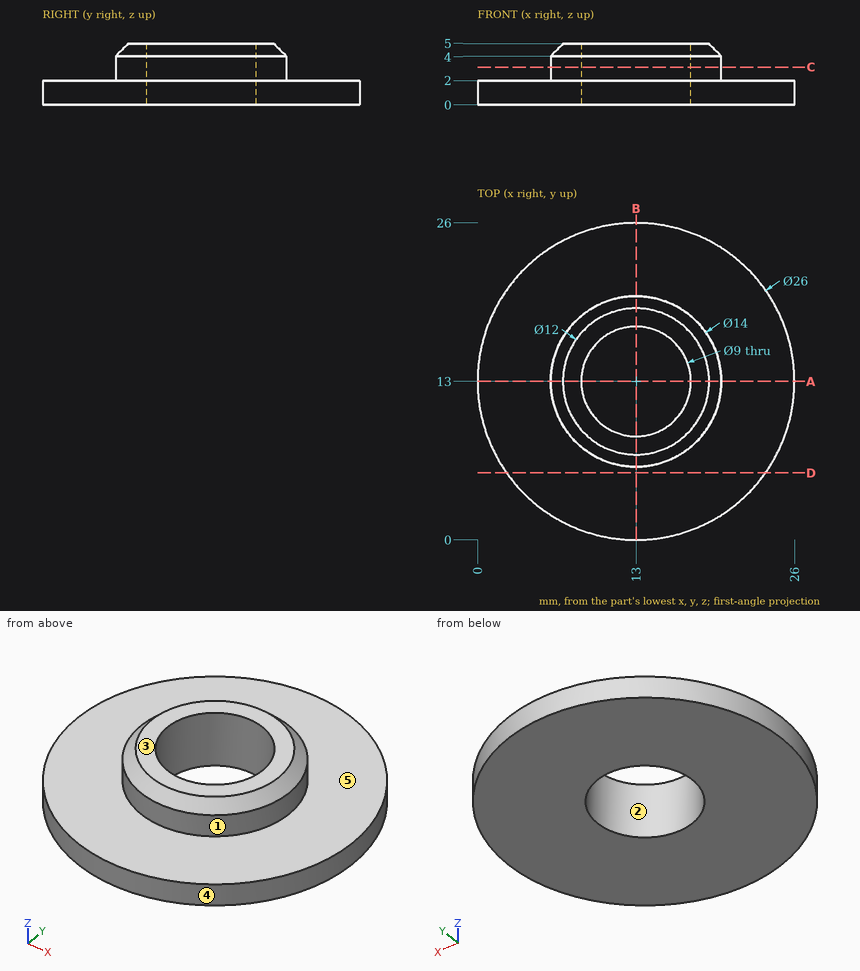
Could you check a few things on this drawing? It's one solid part, dimensions in mm from its lowest x, y, z. A direction names the side the tool comes from. Round coordinates to 2 decimals unless told otherwise and drop trailing zeros. Loops run counter-clockwise (first coordinate to the right, second up) from the corner with the lowest first, then second, coordinate; pieces in that order, holes last.
Q1. Thinking about a two-plate mould opening in X: for the marked faces 1, 2 and 3, which applies, pulls with the +X half, pulls with the -X half, needs draft (parallel to the pull), parting line crosses it, or undercut?
Q2. Please list where these lines run through material, in increasing order: L1, parallel to Y at x = 13, z = 1.45; L2, parallel to Y at x = 13, z = 2.3; L3, parallel to Z at x = 24, y = 19.5.
Q3. On a 3-axis mill with a long thin cutter (end or side, diameter ignored), from which of +Z, -Z, +X, -X, +Y, -Y can I reach the whole of each face in a straight line? I mean the marked faces 4 and 5. Say none if no direction works.
Q4. I want a section at C-C (z = 3.1). Write out the boundary of the cut face in (x, y).
Q5. I want a section at A-A (y = 13). Write out the boundary of the cut face in (x, z).
Q6. For P1, Ø2, axis at y = 10.5, z = 1.5, coming from the -X side, with a flat end and sliding along its axis, tell me the tip position at first contact or that it passes through.
Q7. I want a section at D-D (y = 5.5). Write out the boundary of the cut face in (x, z), and give its area (3 significant figures).
Answer below:
1. face 1: parting line crosses it
1. face 2: undercut
1. face 3: needs draft
2. L1: y = 0 to 8.5, 17.5 to 26
2. L2: y = 6 to 8.5, 17.5 to 20
2. L3: z = 0 to 2
3. face 4: +Z, -Z
3. face 5: +Z
4. outline: circle Ø14 at (13, 13); hole circle Ø9 at (13, 13)
5. outline: (0, 0) - (8.5, 0) - (8.5, 5) - (7, 5) - (6, 4) - (6, 2) - (0, 2) - close; (17.5, 0) - (26, 0) - (26, 2) - (20, 2) - (20, 4) - (19, 5) - (17.5, 5) - close
6. P1: stops at x = 0.09
7. outline: (2.38, 0) - (23.62, 0) - (23.62, 2) - (2.38, 2) - close
7. area: 42.5 mm2
